Build history of the part. All positions in model axes, mm. A direction names the side the tool comes from. Give positions to 0.01 mm unless a question says otherwise; leave off trailing zeros. Order: outer loops, then holes, each group sorted by start corner. A loop starts at its lowest first (then second) coordinate and runs counter-clockwise, first axis right, second up. Notation, with made-up numbers: (78, 84) -> (92, 84) arc R18 cw to (92, 106) -> close; hole circle Ø2 at (-12.5, 40). An arc over 180 degrees is marked (long way). One line per item, written item: value. Start each with the question number.
(1) Two-plate mould, pull along Y, no slides. Class faces 1 (the cylindrical face through (12.57, 2.03, 12)), 2 (the flat face through (-8.22, -8.13, 4.51)), 3 (the flat face through (-1.86, -10.3, -8.79)): +Y half, -Y half, draft (parallel to the pull), parting line (faces both ways), or undercut.
(2) Probe line 1 (X direction, y = 2.95, z = -13.5); line 2 (Z direction, x = -10, y = -5.25); line 3 (Z direction, x = 5.5, y = -5.5). List the from-to ranges inside material, lowest first.
(3) Which spindle directions (+Z, -Z, +X, -X, +Y, -Y) get a long thin tool onto all of the face, cutting with end or side? Do faces 4 (the flat face through (-6.1, -14.8, 3)), 5 (the flat face through (13, -2, -0.75)), 6 (the flat face through (9.75, -13.05, 9.75)), 7 (the flat face through (-3.895, -20.722, 4.507)). Say none if no direction does.
(4) Pin check, flat tips, straight feed: pin 1 (3 mm diameter, centred on x = -4.5, y = -15, fed in from -Z); pin 2 (3 mm diameter, centred on y = 2.5, z = 2.5, fed in from +X); pin 3 (4 mm diameter, centred on x = -4.5, y = -19.5, fed in from -Z). Stop position of each tip, or through.
(5) Saw through at B-B on z = 3. Give the cut face in (x, y).
(6) Saw through at A-A on z = -13.5. Give the cut face in (x, y), plus the area to 3 significant figures.
(7) Saw through at C-C on x = 12.5. Count the separate pieces of the cut face and the enclosed holes in it, plus the area to 3 significant figures.
```python
from build123d import *
from build123d.topology import SkipClean

# Parameters (mm, degrees)
BOSS_EXTRUDE1_DEPTH            = 4
SKETCH2_R                      = 1.5
CUT_EXTRUDE1_DEPTH             = 26.069902273
BOSS_EXTRUDE2_REACH            = 40.332
SKETCH4_R                      = 8
SKETCH5_R                      = 8
CUT_EXTRUDE2_DEPTH             = 20
BOSS_EXTRUDE3_DEPTH            = 0.75
BOSS_EXTRUDE3_DEPTH_BACK       = 0.75
SKETCH8_R                      = 3.5
SKETCH8_R_2                    = 1.5
BOSS_EXTRUDE4_DEPTH            = 4
BOSS_EXTRUDE5_START            = 5
SKETCH9_R                      = 1.5
BOSS_EXTRUDE5_DEPTH            = 5
CUT_EXTRUDE3_REACH             = 39.025
CUT_EXTRUDE3_END_RADIUS        = 8
SKETCH10_W                     = 2
SKETCH10_H                     = 23
CUT_EXTRUDE3_DIRECTION_2_DEPTH = 38.025134912
CUT_EXTRUDE4_DEPTH             = 0.5
CUT_EXTRUDE5_DEPTH             = 40.98829237
CUT_EXTRUDE5_DEPTH_BACK        = 0.5
SKETCH13_R                     = 7.5
CUT_EXTRUDE6_DEPTH             = 34.897839558
CUT_EXTRUDE7_DEPTH             = 1


with BuildPart() as part:
    # Sketch1 → Boss-Extrude1 (new body)
    with BuildSketch(Plane(origin=(0, 0, 0), x_dir=(1, 0, 0), z_dir=(0, 1, 0))):
        Polygon((-17.5, 14.671572875), (-14.671572875, 17.5), (14.671572875, 17.5), (17.5, 14.671572875), (17.5, -14.671572875), (14.671572875, -17.5), (-14.671572875, -17.5), (-17.5, -14.671572875), align=None)
    extrude(amount=BOSS_EXTRUDE1_DEPTH)

    # Sketch2 → Cut-Extrude1 (cut, through all)
    with BuildSketch(Plane(origin=(0, 4, 0), x_dir=(1, 0, 0), z_dir=(0, 1, 0))):
        with Locations(Location((-12.5, 13.5, 0), (0, 0, 270))):
            Circle(SKETCH2_R)
        with Locations(Location((12.5, 13.5, 0), (0, 0, 270))):
            Circle(SKETCH2_R)
        with Locations(Location((-12.5, -13.5, 0), (0, 0, 270))):
            Circle(SKETCH2_R)
        with Locations(Location((12.5, -13.5, 0), (0, 0, 270))):
            Circle(SKETCH2_R)
    extrude(amount=-CUT_EXTRUDE1_DEPTH, mode=Mode.SUBTRACT)

    # Boss-Extrude2: up to this plane
    boss_extrude2_end = Plane(origin=(0, 0, 0), z_dir=(0, 1, 0))
    # Sketch4 → Boss-Extrude2 (add, up to the surface)
    with BuildSketch(Plane(origin=(8.452365235, -18.126155741, 0), x_dir=(-0.906307787036651, -0.42261826174069733, 0), z_dir=(0.4226182617406973, -0.9063077870366509, 0)), mode=Mode.PRIVATE) as boss_extrude2_sk1:
        Polygon((10, 5), (10, -5), (6.91357525, -7.544402143), (5.190195094, -10), (-5.190195094, -10), (-6.91357525, -7.544402143), (-10, -5), (-10, 5), (-6.91357525, 7.544402143), (-5.190195094, 10), (5.190195094, 10), (6.91357525, 7.544402143), align=None)
        with Locations(Location((0, 0, 0), (0, 0, 180))):
            Circle(SKETCH4_R, mode=Mode.SUBTRACT)
    boss_extrude2_tool1 = split(extrude(boss_extrude2_sk1.sketch, amount=-BOSS_EXTRUDE2_REACH, mode=Mode.PRIVATE), bisect_by=boss_extrude2_end, keep=Keep.BOTH, mode=Mode.PRIVATE)
    add(boss_extrude2_tool1.solids().sort_by_distance((-0.35437, -22.232804, 0))[0])

    # Sketch5 → Cut-Extrude2 (cut)
    with SkipClean():  # the faces are left unmerged after this step: merging them gives an invalid solid
        with BuildSketch(Plane(origin=(8.452365235, -18.126155741, 0), x_dir=(-0.906307787036651, -0.42261826174069733, 0), z_dir=(0.4226182617406973, -0.9063077870366509, 0))):
            with Locations(Location((0, 0, 0), (0, 0, 180))):
                Circle(SKETCH5_R)
        extrude(amount=-CUT_EXTRUDE2_DEPTH, mode=Mode.SUBTRACT)

    # Sketch7 → Boss-Extrude3 (add, two sides: drawn at the far end of the back side and taken through both)
    with SkipClean():  # the faces are left unmerged after this step: merging them gives an invalid solid
        with BuildSketch(Plane.XY.offset(-BOSS_EXTRUDE3_DEPTH_BACK)):
            Polygon((11.03377919, 0), (13.831625139, -6), (13.831625139, 0), align=None)
        extrude(amount=BOSS_EXTRUDE3_DEPTH + BOSS_EXTRUDE3_DEPTH_BACK)

    # Sketch8 → Boss-Extrude4 (add)
    # profile 1 of 6: a face of its own
    with SkipClean():  # the faces are left unmerged after this step: merging them gives an invalid solid
        with BuildSketch(Plane.XY):
            with Locations((-10.613601219, -9.182780106)):
                Circle(SKETCH8_R)
            with Locations((-10.613601219, -9.182780106)):
                Circle(SKETCH8_R_2, mode=Mode.SUBTRACT)
        # profile 2 of 6: a face of its own
        with BuildSketch(Plane.XY):
            with BuildLine():
                ThreePointArc((-12.092765136, -6.010702851), (-9.41653072, -5.893855932), (-7.441523967, -7.703616185))
                Line((-7.441523967, -7.703616185), (-8.920687881, -4.531538935))
                Line((-8.920687881, -4.531538935), (-12.092765136, -6.010702851))
            make_face()
        # profile 3 of 6: a face of its own
        with BuildSketch(Plane.XY):
            with BuildLine():
                Line((-9.134437303, -12.354857361), (-5.962360049, -10.875693444))
                Line((-5.962360049, -10.875693444), (-7.441523967, -7.703616185))
                ThreePointArc((-7.441523967, -7.703616185), (-7.196565195, -8.425241454), (-7.113601219, -9.182780106))
                ThreePointArc((-7.113601219, -9.182780106), (-7.661731159, -11.063328735), (-9.134437303, -12.354857361))
            make_face()
        # profile 4 of 6: a face of its own
        with BuildSketch(Plane.XY):
            with Locations((-5.96480034, -19.152165763)):
                Circle(SKETCH8_R)
            with Locations((-5.96480034, -19.152165763)):
                Circle(SKETCH8_R_2, mode=Mode.SUBTRACT)
        # profile 5 of 6: a face of its own
        with BuildSketch(Plane.XY):
            with BuildLine():
                Line((-2.792723069, -17.673001883), (-4.271887002, -14.500924593))
                Line((-4.271887002, -14.500924593), (-7.443964256, -15.980088509))
                ThreePointArc((-7.443964256, -15.980088509), (-4.76772982, -15.863241597), (-2.792723069, -17.673001883))
            make_face()
        # profile 6 of 6: a face of its own
        with BuildSketch(Plane.XY):
            with BuildLine():
                Line((-1.31355917, -20.845079102), (-2.792723069, -17.673001883))
                ThreePointArc((-2.792723069, -17.673001883), (-2.547764311, -18.394627134), (-2.46480034, -19.152165763))
                ThreePointArc((-2.46480034, -19.152165763), (-3.01293028, -21.032714393), (-4.485636424, -22.324243018))
                Line((-4.485636424, -22.324243018), (-1.31355917, -20.845079102))
            make_face()
        extrude(amount=-BOSS_EXTRUDE4_DEPTH)

    # Sketch9 → Boss-Extrude5 (add)
    # profile 1 of 2: a face of its own
    with SkipClean():  # the faces are left unmerged after this step: merging them gives an invalid solid
        with BuildSketch(Plane.XY.offset(BOSS_EXTRUDE5_START)):
            with BuildLine():
                Line((-12.371097281, -5.589563219), (-9.159758839, -4.01884961))
                Line((-9.159758839, -4.01884961), (-5.751050918, -11.328847338))
                Line((-5.751050918, -11.328847338), (-8.923128172, -12.808011254))
                ThreePointArc((-8.923128172, -12.808011254), (-14.22298081, -10.906838971), (-12.371097281, -5.589563219))
            make_face()
            with Locations((-10.613601219, -9.182780106)):
                Circle(SKETCH9_R, mode=Mode.SUBTRACT)
        # profile 2 of 2: a face of its own
        with BuildSketch(Plane.XY.offset(BOSS_EXTRUDE5_START)):
            with BuildLine():
                Line((-7.655273387, -15.526934615), (-4.483196133, -14.047770699))
                Line((-4.483196133, -14.047770699), (-1.102250039, -21.298232995))
                Line((-1.102250039, -21.298232995), (-4.274327293, -22.777396911))
                ThreePointArc((-4.274327293, -22.777396911), (-9.590031488, -20.84263881), (-7.655273387, -15.526934615))
            make_face()
            with Locations((-5.96480034, -19.152165763)):
                Circle(SKETCH9_R, mode=Mode.SUBTRACT)
        extrude(amount=-BOSS_EXTRUDE5_DEPTH)

    # Cut-Extrude3: up to this cylinder (the profile starts outside it)
    cut_extrude3_end = Plane(origin=(3.592255235, -7.703616212, 0), z_dir=(0.4226182617406974, -0.906307787036651, 0)) * Cylinder(CUT_EXTRUDE3_END_RADIUS, 95.05, mode=Mode.PRIVATE)
    # Sketch10 → Cut-Extrude3 (cut, up to the surface)
    with BuildSketch(Plane(origin=(-9.06307787, -4.226182617, 0), x_dir=(0, 0, 1), z_dir=(-0.9063077870366509, -0.42261826174069744, 0)), mode=Mode.PRIVATE) as cut_extrude3_sk1:
        with Locations((0, -8.5)):
            Rectangle(SKETCH10_W, SKETCH10_H)
    cut_extrude3_tool1 = extrude(cut_extrude3_sk1.sketch, amount=-CUT_EXTRUDE3_REACH, mode=Mode.PRIVATE) - cut_extrude3_end
    add(cut_extrude3_tool1.solids().sort_by_distance((-5.470823, -11.929799, 0))[0], mode=Mode.SUBTRACT)

    # Sketch10 → Cut-Extrude3 direction 2 (cut)
    with BuildSketch(Plane(origin=(-9.06307787, -4.226182617, 0), x_dir=(0, 0, 1), z_dir=(-0.9063077870366509, -0.42261826174069744, 0))):
        with Locations((0, -8.5)):
            Rectangle(SKETCH10_W, SKETCH10_H)
    extrude(amount=CUT_EXTRUDE3_DIRECTION_2_DEPTH, mode=Mode.SUBTRACT)

    # Sketch11 → Cut-Extrude4 (cut)
    with BuildSketch(Plane.XY.offset(10)):
        Polygon((3.748451005, -20.319626969), (3.71195746, -11.509620837), (6.430880821, -10.241766052), (13.156279465, -15.932684512), align=None)
    extrude(amount=-CUT_EXTRUDE4_DEPTH, mode=Mode.SUBTRACT)

    # Sketch12 → Cut-Extrude5 (cut, two sides: drawn at the far end of the back side and taken through both)
    with BuildSketch(Plane(origin=(0, 0, -10), x_dir=(-1, 0, 0), z_dir=(0, 0, -1)).offset(-CUT_EXTRUDE5_DEPTH_BACK)):
        Polygon((-6.430880821, -10.241766052), (-13.156279465, -15.932684512), (-3.748451005, -20.319626969), (-3.71195746, -11.509620837), align=None)
    extrude(amount=CUT_EXTRUDE5_DEPTH + CUT_EXTRUDE5_DEPTH_BACK, mode=Mode.SUBTRACT)

    # Sketch13 → Cut-Extrude6 (cut, through all)
    with BuildSketch(Plane(origin=(0, 0, 0), x_dir=(0.9063077870366509, 0.4226182617406975, 0), z_dir=(0.4226182617406975, -0.9063077870366509, 0))):
        Circle(SKETCH13_R)
    extrude(amount=-CUT_EXTRUDE6_DEPTH, mode=Mode.SUBTRACT)

    # Sketch14 → Cut-Extrude7 (cut)
    with BuildSketch(Plane.XY.offset(5)):
        with BuildLine():
            Line((-11.823546576, -6.42656778), (-13.585542494, -8.854606161))
            Line((-13.585542494, -8.854606161), (-12.103562342, -9.009529269))
            ThreePointArc((-12.103562342, -9.009529269), (-11.817319984, -8.287759919), (-11.208542155, -7.805810505))
            Line((-11.208542155, -7.805810505), (-11.823546576, -6.42656778))
        make_face()
        with BuildLine():
            Line((-9.73260326, -7.968760915), (-8.839805697, -6.738481815))
            Line((-8.839805697, -6.738481815), (-11.823546576, -6.42656778))
            Line((-11.823546576, -6.42656778), (-11.208542155, -7.805810505))
            ThreePointArc((-11.208542155, -7.805810505), (-10.448994524, -7.69183925), (-9.73260326, -7.968760915))
        make_face()
        with BuildLine():
            Line((-9.120022184, -9.321422322), (-7.618060736, -9.478434233))
            Line((-7.618060736, -9.478434233), (-8.839805697, -6.738481815))
            Line((-8.839805697, -6.738481815), (-9.73260326, -7.968760915))
            ThreePointArc((-9.73260326, -7.968760915), (-9.27728222, -8.501420046), (-9.113601219, -9.182780106))
            ThreePointArc((-9.113601219, -9.182780106), (-9.11520732, -9.252175518), (-9.120022184, -9.321422322))
        make_face()
        with BuildLine():
            Line((-9.986879383, -10.545578601), (-9.380056654, -11.906472615))
            Line((-9.380056654, -11.906472615), (-7.618060736, -9.478434233))
            Line((-7.618060736, -9.478434233), (-9.120022184, -9.321422322))
            ThreePointArc((-9.120022184, -9.321422322), (-9.38944494, -10.049637305), (-9.986879383, -10.545578601))
        make_face()
        with BuildLine():
            Line((-12.363797533, -11.594558579), (-9.380056654, -11.906472615))
            Line((-9.380056654, -11.906472615), (-9.986879383, -10.545578601))
            ThreePointArc((-9.986879383, -10.545578601), (-10.760903314, -10.675529949), (-11.494599179, -10.396799297))
            Line((-11.494599179, -10.396799297), (-12.363797533, -11.594558579))
        make_face()
        with BuildLine():
            Line((-13.585542494, -8.854606161), (-12.363797533, -11.594558579))
            Line((-12.363797533, -11.594558579), (-11.494599179, -10.396799297))
            ThreePointArc((-11.494599179, -10.396799297), (-11.987097224, -9.785696954), (-12.103562342, -9.009529269))
            Line((-12.103562342, -9.009529269), (-13.585542494, -8.854606161))
        make_face()
        Polygon((-8.944205163, -18.801242837), (-5.96480034, -19.152165763), (-7.150594583, -16.396464035), align=None)
        Polygon((-7.150594583, -16.396464035), (-5.96480034, -19.152165763), (-4.17118976, -16.747386962), align=None)
        Polygon((-4.17118976, -16.747386962), (-5.96480034, -19.152165763), (-2.985395517, -19.50308869), align=None)
        Polygon((-5.96480034, -19.152165763), (-4.779006098, -21.907867491), (-2.985395517, -19.50308869), align=None)
        Polygon((-7.758410921, -21.556944565), (-4.779006098, -21.907867491), (-5.96480034, -19.152165763), align=None)
        Polygon((-7.758410921, -21.556944565), (-5.96480034, -19.152165763), (-8.944205163, -18.801242837), align=None)
    extrude(amount=-CUT_EXTRUDE7_DEPTH, mode=Mode.SUBTRACT)


solid = part.part
```
Results below:
1. face 1: draft
1. face 2: undercut
1. face 3: -Y half
2. line 1: x = -17.5 to -14, -11 to 11, 14 to 17.5
2. line 2: z = -4 to -1, 1 to 5
2. line 3: z = -10 to -7.54, 7.54 to 10
3. face 4: +Z, -Z, -X
3. face 5: -Z, +X
3. face 6: +Z, -Y
3. face 7: +Z
4. pin 1: stops at z = -5.89
4. pin 2: stops at x = 17.5
4. pin 3: stops at z = -4
5. outline: (-17.5, 0) -> (-11.03, 0) -> (-9.16, -4.02) -> (-12.37, -5.59) arc R4 ccw to (-8.92, -12.81) -> (-5.75, -11.33) -> (-4.48, -14.05) -> (-7.66, -15.53) arc R4 ccw to (-4.27, -22.78) -> (-1.1, -21.3) -> (-0.61, -22.35) -> (1.73, -21.26) -> (-8.18, 0) -> (-7.58, 0) -> (-9.45, 4) -> (-17.5, 4) -> close; (5.72, 4) -> (6.23, 2.91) -> (6.72, 3.13) -> (15.17, -14.99) -> (17.52, -13.9) -> (11.03, 0) -> (17.5, 0) -> (17.5, 4) -> close; hole circle Ø3 at (-10.61, -9.18); hole circle Ø3 at (-5.96, -19.15)
6. outline: (-17.5, 0) -> (-14, 0) -> (-14, 4) -> (-17.5, 4) -> close; (-11, 0) -> (11, 0) -> (11, 4) -> (-11, 4) -> close; (14, 0) -> (17.5, 0) -> (17.5, 4) -> (14, 4) -> close
6. area: 116 mm²
7. separate pieces: 3
7. enclosed holes: 0
7. area: 239 mm²
